CAD build for the part. Positions are in the model's coordinates, mm. Coordinates: 2 decimals unless noted, no trailing zeros. Loops run counter-clockwise (first coordinate to the right, second up) from the corner with the lowest first, then second, coordinate; pieces in that order, holes last.
1) Saw through at A-A, the plane x = 15. Write the cut outline in (y, z), and give its area (3 significant figures).
2) Pin check, flat tips, straight feed: pin 1 Ø17 at (y, z) = (1265, 33) entering from +X; pin 2 Ø5 at (y, z) = (1145.5, 12) entering from -X. Stop position of each tip, or through.
3) Wall check: line 1 along Y through (x, z) = (15, 1); line 2 along Z through (x, y) = (16.5, 1726); line 3 along X through (y, z) = (1940, 1.35). Give the ranges that are in metal, low to high.
4) Saw through at B-B, the plane y = 1757. Write the cut outline in (x, z).
5) Two-plate mould, pull along Z, no slides. Class faces 1 (the flat face through (1.33, 1917.71, 33.35)), 2 (the flat face through (0, 961, 25)), 3 (the flat face through (3, 961, 25)): +Z half, -Z half, draft (parallel to the pull), parting line (faces both ways), or undercut.
6) Saw through at C-C, the plane z = 26.5. Write the cut outline in (x, y).
```python
from build123d import *

# Parameters (mm, degrees)
F1_DEPTH = 1950
F3_DEPTH = 25
F5_DEPTH = 25
F6_R     = 6
F7_DEPTH = 3.001
F8_R     = 6.25
F9_DEPTH = 3.001


with BuildPart() as f1:
    # F0 (on Front) → F1 (new body)
    with BuildSketch(Plane.XZ):
        with BuildLine():
            Line((0, 0), (25, 0))
            Line((25, 0), (25, 3))
            Line((25, 3), (8, 3))
            ThreePointArc((8, 3), (4.464466, 4.464466), (3, 8))
            Line((3, 8), (3, 42))
            ThreePointArc((3, 42), (4.464466, 45.535534), (8, 47))
            Line((8, 47), (25, 47))
            Line((25, 47), (25, 50))
            Line((25, 50), (0, 50))
            Line((0, 50), (0, 0))
        make_face()
    extrude(amount=-F1_DEPTH)

    # F2 (on Right) → F3 (cut)
    with BuildSketch(Plane.YZ):
        Polygon((0, 49), (0, 3), (50, 50), (0, 50), align=None)
    extrude(amount=F3_DEPTH, mode=Mode.SUBTRACT)

    # F4 (on face) → F5 (cut)
    with BuildSketch(Plane(origin=(0, 0, 0), x_dir=(0, -1, 0), z_dir=(-1, 0, 0))):
        Polygon((-1950, 3), (-1900, 50), (-1950, 50), align=None)
    extrude(amount=-F5_DEPTH, mode=Mode.SUBTRACT)

    # F6 (on face) → F7 (cut, through all)
    with BuildSketch(Plane.XY.offset(3)):
        with Locations((15, 10)):
            Circle(F6_R)
    extrude(amount=-F7_DEPTH, mode=Mode.SUBTRACT)

    # F8 (on face) → F9 (cut, through all)
    with BuildSketch(Plane.XY.offset(3)):
        with Locations((15, 1940)):
            Circle(F8_R)
    extrude(amount=-F9_DEPTH, mode=Mode.SUBTRACT)


solid = f1.part
```
Data:
1. outline: (0, 0) - (4, 0) - (4, 3) - (0, 3) - close; (16, 0) - (1933.75, 0) - (1933.75, 3) - (16, 3) - close; (46.81, 47) - (1903.19, 47) - (1900, 50) - (50, 50) - close; (1946.25, 0) - (1950, 0) - (1950, 3) - (1946.25, 3) - close
1. area: 11,300 mm2
2. pin 1: stops at x = 3
2. pin 2: stops at x = 0
3. line 1: y = 0 to 4, 16 to 1933.75, 1946.25 to 1950
3. line 2: z = 0 to 3, 47 to 50
3. line 3: x = 0 to 8.75, 21.25 to 25
4. outline: (0, 0) - (25, 0) - (25, 3) - (8, 3) arc R5 cw to (3, 8) - (3, 42) arc R5 cw to (8, 47) - (25, 47) - (25, 50) - (0, 50) - close
5. face 1: +Z half
5. face 2: draft
5. face 3: undercut
6. outline: (0, 25) - (3, 25) - (3, 1925) - (0, 1925) - close
